Verification items for this drawing (mm, ordinates from the low corner). A direction names the side the tool comes from. Round coordinates to 2 decimals unless told otherwise and drop trailing zeros. Order: outer loops, then holes, each group sorted by start corner. A loop starts at its lowest first (then second) coordinate and runs counter-clockwise, first axis right, second up.
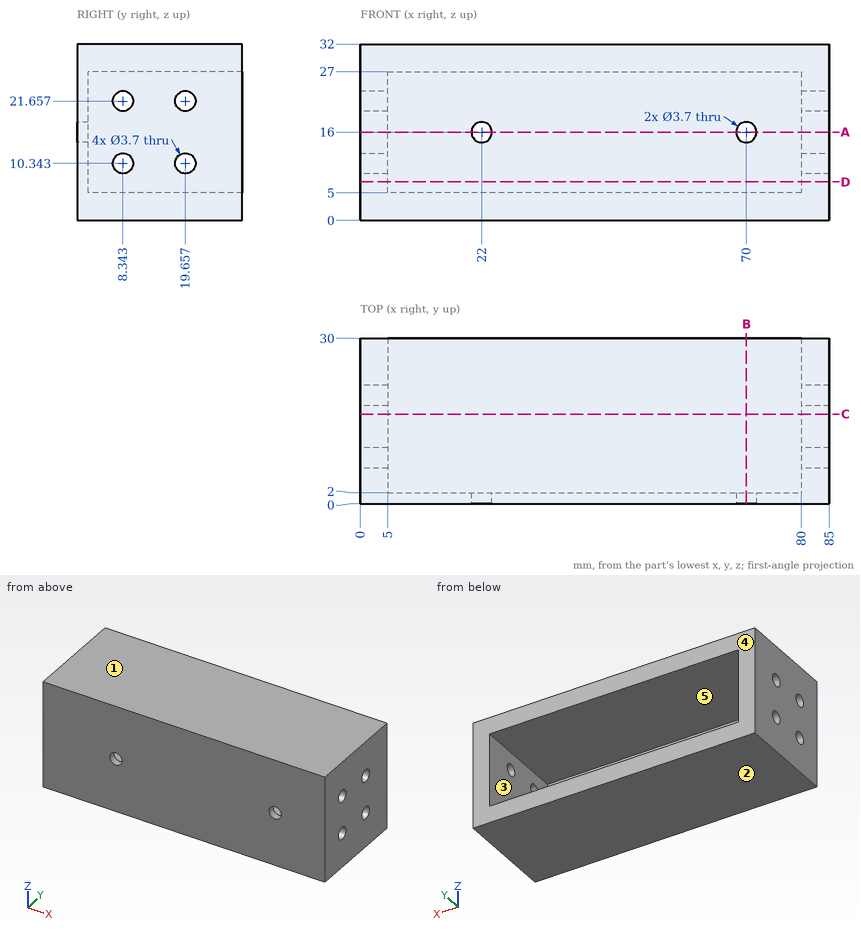
Item 1: Go/stop test with a flat-tipped pin: P1, Ø8, axis at x = 55.5, z = 16.5, coming from the +Y side. Record where the tip stops, or that it passes through.
Answer:
P1: stops at y = 2
Item 2: Sectioned sample at C-C (y = 16.25). Record the cut outline in (x, z), and give its area (3 significant figures).
Answer:
outline: (0, 0) - (85, 0) - (85, 32) - (0, 32) - close; hole (5, 5) - (80, 5) - (80, 27) - (5, 27) - close
area: 1,070 mm2
Item 3: Release check for a two-part mould opening along Z. For the marked faces 1, 2 and 3 record: released by +Z, released by -Z, zero draft, split by the parting line, or undercut.
Answer:
face 1: released by +Z
face 2: released by -Z
face 3: undercut
Item 4: Scan lines: line 1 along X through (y, z) = (8, 24.5); line 2 along Z through (x, y) = (28, 26.5); line 3 along X through (y, z) = (1.5, 14.5). Record each from-to range of solid material in increasing order.
Answer:
line 1: x = 0 to 5, 80 to 85
line 2: z = 0 to 5, 27 to 32
line 3: x = 0 to 20.92, 23.08 to 68.92, 71.08 to 85
Item 5: Sectioned sample at A-A (z = 16). Record the cut outline in (x, y).
Answer:
outline: (0, 0) - (20.15, 0) - (20.15, 2) - (5, 2) - (5, 30) - (0, 30) - close; (23.85, 0) - (68.15, 0) - (68.15, 2) - (23.85, 2) - close; (71.85, 0) - (85, 0) - (85, 30) - (80, 30) - (80, 2) - (71.85, 2) - close
Item 6: Sectioned sample at D-D (z = 7). Record the cut outline in (x, y).
Answer:
outline: (0, 0) - (85, 0) - (85, 30) - (80, 30) - (80, 2) - (5, 2) - (5, 30) - (0, 30) - close
Item 7: Access from +Z, -Z, +X, -X, +Y, -Y to the whole of each face (thin tool, end or side, straight path). Record for the marked faces 4 and 5.
Answer:
face 4: +Z, -Z, +X, -X, +Y
face 5: +Y
Item 8: Sectioned sample at B-B (x = 70). Record the cut outline in (y, z), and give its area (3 significant figures).
Answer:
outline: (0, 0) - (30, 0) - (30, 5) - (2, 5) - (2, 14.15) - (0, 14.15) - close; (0, 17.85) - (2, 17.85) - (2, 27) - (30, 27) - (30, 32) - (0, 32) - close
area: 337 mm2
